from build123d import *

# Parameters (mm, degrees)
EXTRUDE_1_DEPTH     = 36
SKETCH_2_W          = 16.133790568
SKETCH_2_H          = 36
EXTRUDE_2_DEPTH     = 6
EXTRUDE_3_DEPTH     = 36
FILLET_2_R          = 0.5
FILLET_4_R          = 2
CUT_EXTRUDE_START   = -4
CUT_EXTRUDE_1_DEPTH = 4
CUT_EXTRUDE_2_DEPTH = 60.648936936
CUT_EXTRUDE_4_DEPTH = 60.648936936
SKETCH_10_R         = 2
CUT_EXTRUDE_5_DEPTH = 292.913162357
SKETCH_11_R         = 2
EXTRUDE_6_DEPTH     = 1
EXTRUDE_START       = 1
SKETCH_12_R         = 2
EXTRUDE_7_DEPTH     = 1


with BuildPart() as part:
    # 草图1 → 凸台-拉伸1 (new body)
    with BuildSketch(Plane.XY):
        Polygon((299.097748252, 57.483280844), (301.735697168, 22.832042919), (294.730758259, 0), (313.442305989, 11.635922746), (317.295860503, 30.980257384), (315.184988901, 58.707979342), align=None)
    extrude(amount=EXTRUDE_1_DEPTH)

    # 草图2 → 凸台-拉伸2 (add)
    with BuildSketch(Plane(origin=(-2.627453617, 34.513375093, 0), x_dir=(0.9971147561793038, 0.07590891258269725, 0), z_dir=(-0.07590891258269725, 0.9971147561793038, 0))):
        with Locations((310.665166947, -18)):
            Rectangle(SKETCH_2_W, SKETCH_2_H)
    extrude(amount=EXTRUDE_2_DEPTH)

    # 草图3 → 凸台-拉伸3 (add)
    with BuildSketch(Plane.XY.offset(36)):
        Polygon((298.642294776, 63.465969381), (301.735697168, 22.832042919), (294.730758259, 0), (291.40566003, -2.067738419), (298.7443529, 22.604316182), (295.650950508, 63.238242643), align=None)
    extrude(amount=-EXTRUDE_3_DEPTH)

    # 圆角2
    fillet_2_edges = [part.edges().sort_by_distance(p)[0] for p in [
        (291.40566003, -2.067738419, 18),
    ]]
    fillet(fillet_2_edges, radius=FILLET_2_R)

    # 圆角4
    fillet_4_edges = [part.edges().sort_by_distance(p)[0] for p in [
        (317.295860503, 30.980257384, 18),
        (313.442305989, 11.635922746, 18),
        (314.729535426, 64.690667879, 18),
        (298.7443529, 22.604316182, 18),
        (295.650950508, 63.238242643, 18),
    ]]
    fillet(fillet_4_edges, radius=FILLET_4_R)

    # 草图4 → 切除-拉伸1 (cut)
    with BuildSketch(Plane.XY.offset(31).offset(CUT_EXTRUDE_START)):
        with BuildLine():
            Line((292.524622126, -1.371903061), (312.706326829, 11.178248331))
            ThreePointArc((312.706326829, 11.178248331), (313.294550919, 11.738215234), (313.61162859, 12.485899834))
            Line((313.61162859, 12.485899834), (317.242267225, 30.711226207))
            ThreePointArc((317.242267225, 30.711226207), (317.277169716, 30.981386297), (317.27503737, 31.253783271))
            Line((317.27503737, 31.253783271), (314.881353251, 62.696438367))
            ThreePointArc((314.881353251, 62.696438367), (314.189905536, 64.062105166), (312.735305913, 64.538850054))
            Line((312.735305913, 64.538850054), (297.64518002, 63.390060468))
            ThreePointArc((297.64518002, 63.390060468), (296.27951322, 62.698612754), (295.802768333, 61.244013131))
            Line((295.802768333, 61.244013131), (298.716326749, 22.972458573))
            ThreePointArc((298.716326749, 22.972458573), (298.710751525, 22.607910585), (298.639090177, 22.250431957))
            Line((298.639090177, 22.250431957), (291.781334489, -0.804753178))
            ThreePointArc((291.781334489, -0.804753178), (291.957278491, -1.344805743), (292.524622126, -1.371903061))
        make_face()
        with BuildLine():
            Line((312.811214826, 63.541735298), (297.721088933, 62.392945712))
            ThreePointArc((297.721088933, 62.392945712), (297.038255533, 62.047221855), (296.799883089, 61.319922043))
            Line((296.799883089, 61.319922043), (299.713441505, 23.048367486))
            ThreePointArc((299.713441505, 23.048367486), (299.705078669, 22.501545504), (299.597586647, 21.965327561))
            Line((299.597586647, 21.965327561), (293.115505419, 0.173127667))
            Line((293.115505419, 0.173127667), (312.178248026, 12.027443702))
            ThreePointArc((312.178248026, 12.027443702), (312.472360071, 12.307427153), (312.630898906, 12.681269453))
            Line((312.630898906, 12.681269453), (316.261537541, 30.906595826))
            ThreePointArc((316.261537541, 30.906595826), (316.278988787, 31.041675872), (316.277922614, 31.177874358))
            Line((316.277922614, 31.177874358), (313.884238495, 62.620529454))
            ThreePointArc((313.884238495, 62.620529454), (313.538514637, 63.303362854), (312.811214826, 63.541735298))
        make_face(mode=Mode.SUBTRACT)
    cut_extrude_1 = extrude(amount=CUT_EXTRUDE_1_DEPTH, mode=Mode.SUBTRACT)

    # 镜向1: 切除-拉伸1 across plane
    add(cut_extrude_1.mirror(Plane.XY.offset(18)), mode=Mode.SUBTRACT)

    # 草图5 → 切除-拉伸2 (cut, through all)
    with BuildSketch(Plane(origin=(316.815327762, 24.118695337, 0), x_dir=(0, 0, -1), z_dir=(0.9971147561793037, 0.07590891258269838, 0))):
        Polygon((-9, 29.005921915), (-5, 29.005921915), (-5, 7.07960541), (-5, 1.984059182), (-9, 1.984059182), (-9, 7.07960541), align=None)
        with BuildLine():
            Line((-31, 29.005921915), (-31, 7.07960541))
            Line((-31, 7.07960541), (-31, 1.327664424))
            ThreePointArc((-31, 1.327664424), (-29.000294628, 1.441652043), (-27, 1.544783774))
            Line((-27, 1.544783774), (-27, 7.07960541))
            Line((-27, 7.07960541), (-27, 29.005921915))
            Line((-27, 29.005921915), (-31, 29.005921915))
        make_face()
    extrude(amount=-CUT_EXTRUDE_2_DEPTH, mode=Mode.SUBTRACT)

    # 草图9 → 切除-拉伸4 (cut, through all)
    with BuildSketch(Plane(origin=(316.815327762, 24.118695337, 0), x_dir=(0, 0, -1), z_dir=(0.9971147561793037, 0.07590891258269838, 0))):
        Polygon((-9, 38.613242737), (-9, 41.460309821), (-5, 41.460309821), (-5, 38.613242737), (-5, 29.005921915), (-9, 29.005921915), align=None)
        Polygon((-31, 38.613242737), (-31, 44.422842446), (-27, 44.422842446), (-27, 38.613242737), (-27, 29.005921915), (-31, 29.005921915), align=None)
    extrude(amount=-CUT_EXTRUDE_4_DEPTH, mode=Mode.SUBTRACT)

    # 草图10 → 切除-拉伸5 (cut, through all)
    with BuildSketch(Plane(origin=(66.866773871, -81.092277049, 36), x_dir=(0.7883945685937017, 0.6151698986556081, 0), z_dir=(0, 0, 1))):
        with Locations(Location((264.00053068, -51.596816089, 0), (0, 0, 322.035733535))):
            Circle(SKETCH_10_R)
        with Locations(Location((271.852922924, -41.244744086, 0), (0, 0, 322.035733535))):
            Circle(SKETCH_10_R)
    extrude(amount=-CUT_EXTRUDE_5_DEPTH, mode=Mode.SUBTRACT)

    # 草图11 → 凸台-拉伸6 (add)
    with BuildSketch(Plane.XY.offset(27)):
        with BuildLine():
            Line((312.735305913, 64.538850054), (297.64518002, 63.390060468))
            ThreePointArc((297.64518002, 63.390060468), (296.27951322, 62.698612754), (295.802768333, 61.244013131))
            Line((295.802768333, 61.244013131), (298.716326749, 22.972458573))
            ThreePointArc((298.716326749, 22.972458573), (298.710751525, 22.607910585), (298.639090177, 22.250431957))
            Line((298.639090177, 22.250431957), (291.781334489, -0.804753178))
            ThreePointArc((291.781334489, -0.804753178), (291.957278491, -1.344805743), (292.524622126, -1.371903061))
            Line((292.524622126, -1.371903061), (312.706326829, 11.178248331))
            ThreePointArc((312.706326829, 11.178248331), (313.294550919, 11.738215234), (313.61162859, 12.485899834))
            Line((313.61162859, 12.485899834), (317.242267225, 30.711226207))
            ThreePointArc((317.242267225, 30.711226207), (317.277169716, 30.981386297), (317.27503737, 31.253783271))
            Line((317.27503737, 31.253783271), (314.881353251, 62.696438367))
            ThreePointArc((314.881353251, 62.696438367), (314.189905536, 64.062105166), (312.735305913, 64.538850054))
        make_face()
        with Locations((306.74416649, 40.634253093)):
            Circle(SKETCH_11_R, mode=Mode.SUBTRACT)
        with Locations((306.5666668, 53.626325775)):
            Circle(SKETCH_11_R, mode=Mode.SUBTRACT)
    extrude(amount=EXTRUDE_6_DEPTH)

    # 草图12 → 凸台-拉伸7 (add)
    with BuildSketch(Plane(origin=(0, 0, 9), x_dir=(-1, 0, 0), z_dir=(0, 0, -1)).offset(EXTRUDE_START)):
        with BuildLine():
            Line((-298.716326749, 22.972458573), (-295.802768333, 61.244013131))
            ThreePointArc((-295.802768333, 61.244013131), (-296.27951322, 62.698612754), (-297.64518002, 63.390060468))
            Line((-297.64518002, 63.390060468), (-312.735305913, 64.538850054))
            ThreePointArc((-312.735305913, 64.538850054), (-314.189905536, 64.062105166), (-314.881353251, 62.696438367))
            Line((-314.881353251, 62.696438367), (-317.27503737, 31.253783271))
            ThreePointArc((-317.27503737, 31.253783271), (-317.277169716, 30.981386297), (-317.242267225, 30.711226207))
            Line((-317.242267225, 30.711226207), (-313.61162859, 12.485899834))
            ThreePointArc((-313.61162859, 12.485899834), (-313.294550919, 11.738215234), (-312.706326829, 11.178248331))
            Line((-312.706326829, 11.178248331), (-292.524622126, -1.371903061))
            ThreePointArc((-292.524622126, -1.371903061), (-291.957278491, -1.344805743), (-291.781334489, -0.804753178))
            Line((-291.781334489, -0.804753178), (-298.639090177, 22.250431957))
            ThreePointArc((-298.639090177, 22.250431957), (-298.710751525, 22.607910585), (-298.716326749, 22.972458573))
        make_face()
        with Locations(Location((-306.74416649, 40.634253093, 0), (0, 0, 180))):
            Circle(SKETCH_12_R, mode=Mode.SUBTRACT)
        with Locations(Location((-306.5666668, 53.626325775, 0), (0, 0, 180))):
            Circle(SKETCH_12_R, mode=Mode.SUBTRACT)
    extrude(amount=-EXTRUDE_7_DEPTH)


solid = part.part
Source: CAD feature listing. Evaluate the final solid. Frame: model axes, mm. A direction names the side the tool comes from. Round coordinates to 2 decimals unless told otherwise and drop trailing zeros. Loops run counter-clockwise (first coordinate to the right, second up) from the corner with the lowest first, then second, coordinate; pieces in that order, holes last. Notation, with made-up numbers: M 43,-40 L 93,-40 A8 ccw 93,-36 Z; hole C 55,79 d8. An arc over 180 degrees is marked long. Return JSON: item names as keys, results as strings. Group by question number.
1. Pin query (flat end, axial travel): pin 1 (3.5 mm diameter, centred on x = 306.74, y = 40.63, fed in from -Z); pin 2 (1.5 mm diameter, centred on y = 20, z = 4, fed in from +X); pin 3 (1 mm diameter, centred on y = 40.5, z = 12.5, fed in from -X); pin 4 (1 mm diameter, centred on x = 312.5, z = 23, fed in from -Y). Return the tip coordinate at first contact, or that it passes through.
2. Section query A-A on y = 57. Output: boundary loops of the cut face in (x, z).
3. Mould query, pull axis Z, two halves, no side actions, for faces 1 (the face through (299.646, 23.935, 6.521)), 2 (the face through (308.414, 52.86, 33.535)). Classes: released by +Z, released by -Z, zero draft, split by the parting line, or undercut.
4. Section query B-B on z = 21. Output: boundary loops of the cut face in (x, y).
5. Reachability of faces 3 (the face through (302.513, 6.017, 6.521)), 4 (the face through (305.27, 41.986, 2.535)), 5 (the face through (295.16, 10.56, 33.53)), 6 (the face through (307.52, 24.83, 29.52)), 7 (the face through (299.665, 23.687, 29.479)) from +Z, -Z, +X, -X, +Y, -Y: full face, straight path, thin tool, end or side. Return the list, or none.
6. Material intervals for line 1 along Z through (x, y) = (304.5, 54.5); line 2 along Z through (x, y) = (301, 24.5); line 3 along Y through (x, z) = (308, 24), sorted ascending. Write a range as from..to.
7. Section query D-D on y = 13.5. Output: boundary loops of the cut face in (x, z).
8. Section query C-C on y = 3. Output: boundary loops of the cut face in (x, z), and give its area (3 significant figures).
Checks:
{
 "1": {"pin 1": "passes through", "pin 2": "stops at x = 315.26", "pin 3": "stops at x = 297.34", "pin 4": "stops at y = 10.74"},
 "2": {"outline": "M 296.13,0 L 315.32,0 L 315.32,5 L 296.13,5 Z; M 296.13,8 L 315.32,8 L 315.32,28 L 296.13,28 Z; M 296.13,31 L 315.32,31 L 315.32,36 L 296.13,36 Z"},
 "3": {"face 1": "undercut", "face 2": "zero draft"},
 "4": {"outline": "M 291.78,-0.8 A0.5 ccw 292.52,-1.37 L 312.71,11.18 A2 ccw 313.61,12.49 L 317.24,30.71 A2 ccw 317.28,31.25 L 314.88,62.7 A2 ccw 312.74,64.54 L 297.65,63.39 A2 ccw 295.8,61.24 L 298.72,22.97 A2 cw 298.64,22.25 Z; hole C 306.57,53.63 d4; hole C 306.74,40.63 d4"},
 "5": {"face 3": "+X, -Y", "face 4": "+Z, -Z", "face 5": "+Z, -Z, -X", "face 6": "-X, +Y", "face 7": "-X"},
 "6": {"line 1": "z = 0..5, 8..28, 31..36", "line 2": "z = 0..28, 31..36", "line 3": "y = 8.25..39.08, 42.19..52.23, 55.02..64.18"},
 "7": {"outline": "M 296.04,0 L 313.81,0 L 313.81,5 L 312.79,5 L 312.79,8 L 313.81,8 L 313.81,28 L 312.79,28 L 312.79,31 L 313.81,31 L 313.81,36 L 296.04,36 L 296.04,31 L 297.08,31 L 297.08,28 L 296.04,28 L 296.04,8 L 297.08,8 L 297.08,5 L 296.04,5 Z"},
 "8": {"outline": "M 292.91,0 L 299.56,0 L 299.56,5 L 297.66,5 L 297.66,8 L 299.56,8 L 299.56,28 L 297.66,28 L 297.66,31 L 299.56,31 L 299.56,36 L 292.91,36 L 292.91,31 L 293.96,31 L 293.96,28 L 292.91,28 L 292.91,8 L 293.96,8 L 293.96,5 L 292.91,5 Z", "area": "221 mm²"}
}
